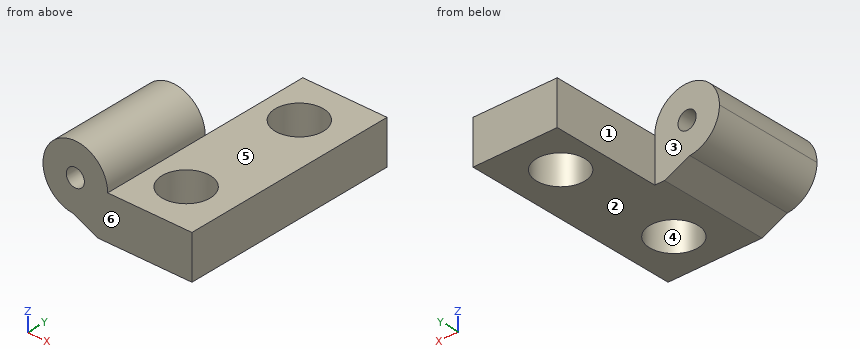
from build123d import *

# Parameters (mm, degrees)
F0_W           = 16
F0_H           = 15
F0_R           = 1.65
F1_DEPTH       = 3
F2_R           = 2.2197148543
F3_DEPTH       = 15
F4_R           = 0.622015
F5_DEPTH       = 25
F7_DEPTH       = 25
F9_DEPTH       = 15
F10_W          = 7.79368474
F10_H          = 8.6547567695
F11_DEPTH      = 25
F11_DEPTH_BACK = 25


with BuildPart() as f1:
    # F0 (on Top) → F1 (new body)
    with BuildSketch(Plane.XY):
        with Locations((8, 7.5)):
            Rectangle(F0_W, F0_H)
        with Locations((3.0942130834, 3.1138566653)):
            Circle(F0_R, mode=Mode.SUBTRACT)
        with Locations((12.8244230834, 3.1138566653)):
            Circle(F0_R, mode=Mode.SUBTRACT)
        with Locations((3.0942130834, 11.8174366653)):
            Circle(F0_R, mode=Mode.SUBTRACT)
        with Locations((12.8244230834, 11.8174366653)):
            Circle(F0_R, mode=Mode.SUBTRACT)
    extrude(amount=F1_DEPTH)

    # F2 (on face) → F3 (join, through all)
    with BuildSketch(Plane(origin=(0, 15, 0), x_dir=(-1, 0, 0), z_dir=(0, 1, 0))):
        with Locations((-8, 3)):
            Circle(F2_R)
    extrude(amount=-F3_DEPTH)

    # F4 (on face) → F5 (cut)
    with BuildSketch(Plane(origin=(0, 15, 0), x_dir=(-1, 0, 0), z_dir=(0, 1, 0))):
        with Locations((-8, 3)):
            Circle(F4_R)
        Polygon((-8, 0.8955585654), (-9.5511529364, 0), (-6.4488470636, 0), align=None)
    extrude(amount=-F5_DEPTH, mode=Mode.SUBTRACT)

    # F6 (on face) → F7 (cut)
    with BuildSketch(Plane(origin=(0, 15, 0), x_dir=(-1, 0, 0), z_dir=(0, 1, 0))):
        with BuildLine():
            ThreePointArc((-5.7802851457, 3), (-6.4976685136, 1.3659454907), (-8.1861204126, 0.7881018951))
            Line((-8.1861204126, 0.7881018951), (-9.5511529364, 0))
            Line((-9.5511529364, 0), (0, -1.0680041742))
            Line((0, -1.0680041742), (0, 3))
            Line((0, 3), (-5.7802851457, 3))
        make_face()
    extrude(amount=-F7_DEPTH, mode=Mode.SUBTRACT)

    # F8 (on face) → F9 (join, through all)
    with BuildSketch(Plane(origin=(0, 15, 0), x_dir=(-1, 0, 0), z_dir=(0, 1, 0))):
        Polygon((-8, 0.8955585654), (-9.5511529364, 0), (-7.8138795874, 0.7881018951), align=None)
    extrude(amount=-F9_DEPTH)

    # F10 (on face) → F11 (cut, two sides)
    with BuildSketch(Plane.XY.offset(3)) as f11_sk:
        with Locations((6.3228724843, 11.8273783848)):
            Rectangle(F10_W, F10_H)
    extrude(amount=-F11_DEPTH, mode=Mode.SUBTRACT)
    extrude(f11_sk.sketch, amount=F11_DEPTH_BACK, mode=Mode.SUBTRACT)


solid = f1.part
Part model, mm, in its own coordinate system. Face numbers are marked on the shaded views. A direction names the side the tool comes from. Give positions to 0.01 mm unless a question says otherwise; leave off trailing zeros. Order: outer loops, then holes, each group sorted by start corner. A loop starts at its lowest first (then second) coordinate and runs counter-clockwise, first axis right, second up. Notation, with made-up numbers: (-36.75, 56) -> (-7.75, 56) arc R21 cw to (-7.75, 94) -> close; hole circle Ø2 at (-18, 45). An arc over 180 degrees is marked (long way). Use one line per item in the form item = value.
(1) Flat gauge pins, fed straight in: P1, Ø5.5, axis at x = 12.82, y = 11.82, coming from the +Z side; P2, Ø1, axis at y = 11, z = 2, coming from the -X side; P3, Ø1.4, axis at x = 8, z = 3, coming from the +Y side. Where does each tip first touch, or does it go through?
Solution:
P1 = 3
P2 = 10.22
P3 = 7.5
(2) Saw through at B-B (x = 13). Write the cut outline in (y, z), then the cut area to 3 significant figures.
Solution:
outline = (0, 0) -> (1.47, 0) -> (1.47, 3) -> (0, 3) -> close; (4.75, 0) -> (10.18, 0) -> (10.18, 3) -> (4.75, 3) -> close; (13.46, 0) -> (15, 0) -> (15, 3) -> (13.46, 3) -> close
area = 25.3 mm²
(3) Saw through at A-A (y = 7). Write the cut outline in (x, z), then the cut area to 3 significant figures.
Solution:
outline = (7.81, 0.79) -> (9.55, 0) -> (16, 0) -> (16, 3) -> (10.22, 3) arc R2.22 ccw (long way) to start; hole circle Ø1.24 at (8, 3)
area = 33.9 mm²
(4) Pull direction Y, two halves, no side cores. Call the marked faces 3, 4, 5 and 6: +Y half, -Y half, draft (parallel to the pull), parting line (faces both ways), or undercut.
Solution:
face_3 = +Y half
face_4 = undercut
face_5 = draft
face_6 = -Y half
(5) Drill centre lines: line 1 (Y direction, x = 13.75, z = 2.65); line 2 (Y direction, x = 13, z = 2.25); line 3 (Z direction, x = 15.5, y = 8). Where is each one in solid material? Low to high. Write a range as from..to.
Solution:
line_1 = 0..1.75, 4.48..10.45, 13.18..15
line_2 = 0..1.47, 4.75..10.18, 13.46..15
line_3 = 0..3
(6) Tool access for the marked faces 1 and 2: list every direction of +Z, -Z, +X, -X, +Y, -Y with a clear straight run to the whole face (end or side of a thin tool).
Solution:
face_1 = +Z, -Z, -X, +Y
face_2 = -Z, +X, -X, +Y, -Y
(7) Saw through at C-C (z = 3.2). Write the cut outline in (x, y).
Solution:
outline = (5.79, 0) -> (7.41, 0) -> (7.41, 7.5) -> (5.79, 7.5) -> close; (8.59, 0) -> (10.21, 0) -> (10.21, 7.5) -> (8.59, 7.5) -> close
(8) Saw through at D-D (y = 10.5). Write the cut outline in (x, z).
Solution:
outline = (10.22, 0) -> (11.83, 0) -> (11.83, 3) -> (10.22, 3) -> close; (13.82, 0) -> (16, 0) -> (16, 3) -> (13.82, 3) -> close
